Work out the finished part from the listing and answer in its coordinate system (mm). Coordinates: 2 decimals unless noted, no trailing zeros. Write each loop counter-clockwise with the first axis right and the second up, starting at its lowest first coordinate (ties: lowest second). Pieces come first, ordered by that corner, then holes. Notation, with made-up numbers: M 63,-33 L 78,-33 A25 cw 78,-12 Z; hole C 57.25,67 d7. An arc over 180 degrees is marked long. Answer as CSV lines item,"result". Start each with the question number.
(1) The mould has two halves that part along Y. Classify faces 1 (the flat face through (0, 150, 0)), 2 (the flat face through (0, 0, 0)), 3 (the cylindrical face through (1.11, 5.88, 0.02)), 4 (the flat face through (0, 68, 0)): released by +Y, released by -Y, zero draft, split by the parting line, or undercut.
(2) Find the intervals of material crossed by L1, parallel to Y at x = 0, z = -0.3; L2, parallel to X at y = 11, z = -0.15; L3, parallel to Y at x = 0.7, z = -0.75, in increasing order. Write a range as [from, to].
(3) A cutting plane is placed at A-A on x = 0. Give the vertices of the cut face in (y, z).
(4) A cutting plane is placed at C-C on y = 139.5. Give the vertices of the cut face in (x, z).
(5) Flat-ended cylindrical pins translate along their axes: P1, Ø0.7, axis at y = 53, z = -0.5, coming from the +X side; P2, Ø0.5, axis at y = 45, z = -0.5, coming from the -X side; P3, Ø1.2, axis at x = 0, y = 56, coming from the -Z side. Find the tip coordinate at first contact, or state that the pin passes through.
(6) A cutting plane is placed at B-B on y = 51.5. Give the vertices of the cut face in (x, z), then the cut area to 3 significant figures.
from build123d import *

# Parameters (mm, degrees)
SKETCH_1_R          = 1.5
EXTRUDE_1_DEPTH     = 150
SKETCH_3_R          = 1.2
CUT_EXTRUDE_2_DEPTH = 150
CUT_EXTRUDE_3_DEPTH = 10


with BuildPart() as part:
    # 草图1 → 凸台-拉伸1 (new body)
    with BuildSketch(Plane(origin=(0, 0, 0), x_dir=(1, 0, 0), z_dir=(0, 1, 0))):
        with Locations(Location((0, 0, 0), (0, 0, 270))):
            Circle(SKETCH_1_R)
    extrude(amount=EXTRUDE_1_DEPTH)

    # 草图3 → 切除-拉伸2 (cut, symmetric)
    with BuildSketch(Plane.XY):
        with Locations((0, 6.338597252)):
            Circle(SKETCH_3_R)
    extrude(amount=CUT_EXTRUDE_2_DEPTH, both=True, mode=Mode.SUBTRACT)

    # 草图5 → 切除-拉伸3 (cut)
    with BuildSketch(Plane.XY):
        with BuildLine():
            Line((1.2, 123.985472487), (1.2, 10.930622971))
            ThreePointArc((1.2, 10.930622971), (0, 9.730622971), (-1.2, 10.930622971))
            Line((-1.2, 10.930622971), (-1.2, 123.985472487))
            ThreePointArc((-1.2, 123.985472487), (0, 125.185472487), (1.2, 123.985472487))
        make_face()
    extrude(amount=-CUT_EXTRUDE_3_DEPTH, mode=Mode.SUBTRACT)


solid = part.part
Here are the results:
1,face 1,"released by +Y"
1,face 2,"released by -Y"
1,face 3,"undercut"
1,face 4,"undercut"
2,L1,"y = [0, 5.14], [7.54, 9.73], [125.19, 150]"
2,L2,"x = [-1.49, -1.2], [1.2, 1.49]"
2,L3,"y = [0, 5.36], [7.31, 9.96], [124.96, 150]"
3,outline,"M 0,-1.5 L 5.14,-1.5 L 5.14,1.5 L 0,1.5 Z; M 7.54,-1.5 L 9.73,-1.5 L 9.73,0 L 125.19,0 L 125.19,-1.5 L 150,-1.5 L 150,1.5 L 7.54,1.5 Z"
4,outline,"C 0,0 d3"
5,P1,"stops at x = 1.49"
5,P2,"stops at x = -1.48"
5,P3,"stops at z = 0"
6,outline,"M -1.2,-0.9 L -1.2,0 L 1.2,0 L 1.2,-0.9 A1.5 ccw long Z"
6,area,"3.90 mm^2"
